The model under review builds one solid part; all positions refer to its coordinate system, in mm. A direction names the side the tool comes from. Give positions to 0.01 mm unless a question says otherwise; leave off trailing zeros. Write each loop counter-clockwise with the first axis right and the second up, starting at its lowest first coordinate (ties: lowest second). Pieces come first, ordered by that corner, then holes.
from build123d import *

# Parameters (mm, degrees)
SKETCH1_W           = 82
SKETCH1_H           = 63
BOSS_EXTRUDE1_DEPTH = 25
SKETCH2_R           = 17
BOSS_EXTRUDE2_DEPTH = 35
SCALE1_SCALE        = 0.1


with BuildPart() as part:
    # Sketch1 → Boss-Extrude1 (new body)
    with BuildSketch(Plane(origin=(0, 0, 0), x_dir=(1, 0, 0), z_dir=(0, 1, 0))):
        with Locations((2.928571429, -13.287946429)):
            Rectangle(SKETCH1_W, SKETCH1_H)
    extrude(amount=BOSS_EXTRUDE1_DEPTH)

    # Sketch2 → Boss-Extrude2 (add)
    with BuildSketch(Plane(origin=(0, 25, 0), x_dir=(1, 0, 0), z_dir=(0, 1, 0))):
        with Locations(Location((-2.071428571, -13.287946429, 0), (0, 0, 270))):
            Circle(SKETCH2_R)
    extrude(amount=BOSS_EXTRUDE2_DEPTH)


with BuildPart() as part_1:
    # Scale1: scaled about (1.941255183, 18.423897472, 13.287946429)
    add(part.part.scale(SCALE1_SCALE).moved(Location((1.747129665, 16.581507725, 11.959151786))))


solid = part_1.part
1) Consider section D-D, the plane x = 5. Give the boundary of the cut face in (y, z).
2) Consider section B-B, the plane x = 0.5. Give the boundary of the cut face in (y, z).
3) Consider section A-A, the plane z = 12. Give the boundary of the cut face in (x, y).
4) To check wall thickness, follow probe 1 along Y at (x, z) = (5.5, 16); probe 2 along X at (y, z) = (21.15, 13); probe 3 along Z at (x, y) = (0, 20.3). State the ranges of each line that lie inside material, in increasing order.
5) Tool access review of faces 1 (the flat face through (2, 18, 10.138)), 2 (the cylindrical face through (1.61, 20.81, 11.59)): name each direction out of +Z, -Z, +X, -X, +Y, -Y from which nothing blocks a thin tool from reaching the whole face with its end or side.
6) Insertion check: pin 1 (1.5 mm diameter, centred on x = 3.5, y = 21.5, fed in from +Z); pin 2 (2 mm diameter, centred on y = 20.5, z = 11, fed in from -X); pin 3 (1.5 mm diameter, centred on y = 22, z = 12.5, fed in from -X). Each pin has a flat end and moves straight along its axis. Give the tip position at first contact, or say it passes through.
7) Consider section C-C, the plane y = 21.6. Give the boundary of the cut face in (x, z).
Answer block:
1. outline: (16.58, 10.14) - (19.08, 10.14) - (19.08, 16.44) - (16.58, 16.44) - close
2. outline: (16.58, 10.14) - (19.08, 10.14) - (19.08, 11.94) - (22.58, 11.94) - (22.58, 14.63) - (19.08, 14.63) - (19.08, 16.44) - (16.58, 16.44) - close
3. outline: (-2.06, 16.58) - (6.14, 16.58) - (6.14, 19.08) - (2.65, 19.08) - (2.65, 22.58) - (0.43, 22.58) - (0.43, 19.08) - (-2.06, 19.08) - close
4. probe 1: y = 16.58 to 19.08
4. probe 2: x = -0.14 to 3.22
4. probe 3: z = 12.57 to 14.01
5. face 1: -Z, +X, -X, +Y, -Y
5. face 2: +Y
6. pin 1: stops at z = 14.48
6. pin 2: stops at x = 0.43
6. pin 3: stops at x = -0.16
7. outline: circle Ø3.4 at (1.54, 13.29)
